Check sheet for the modelled part. Datum: model origin and axes. Units: mm. Coordinates: 2 decimals unless noted, no trailing zeros. Write each loop counter-clockwise with the first axis right and the second up, starting at its lowest first coordinate (ties: lowest second). Pieces come first, ordered by that corner, then holes. Notation, with made-up numbers: (-36, 71) - (20, 71) arc R20 cw to (20, 95) - close; hole circle Ø3 at (31.5, 89). An arc over 180 degrees is marked (long way). Use one line per item in the form item = value. Start each with the question number.
1. Cross-section at A-A on z = 15. Record the boundary of the cut face in (x, y) (3 decimals), then the cut area to 3 significant figures.
2. Cross-section at B-B on x = 12. Record the boundary of the cut face in (y, z).
3. Cross-section at D-D on y = 0.7. Give the number of separate pieces and of enclosed holes in the cut face, then the cut area to 3 significant figures.
4. Go/stop test with flat-tipped pins: pin 1 Ø4.5 at (x, z) = (-31, 0) entering from +Y; pin 2 Ø0.5 at (y, z) = (0.5, -0.5) entering from +X; pin 3 Ø0.5 at (y, z) = (0.5, -4) entering from -X; pin 4 Ø0.8 at (y, z) = (0.5, 3.5) entering from -X. Record where each tip stops, or that it passes through.
5. Scan lines: line 1 along X through (y, z) = (0.75, -15) (3 decimals); line 2 along X through (y, z) = (1.1, -7.5); line 3 along Z through (x, y) = (-4.5, 1.65). Record each from-to range of solid material in increasing order.
6. Cross-section at C-C on z = 0. Record the boundary of the cut face in (x, y) (3 decimals), then the cut area to 4 significant figures.
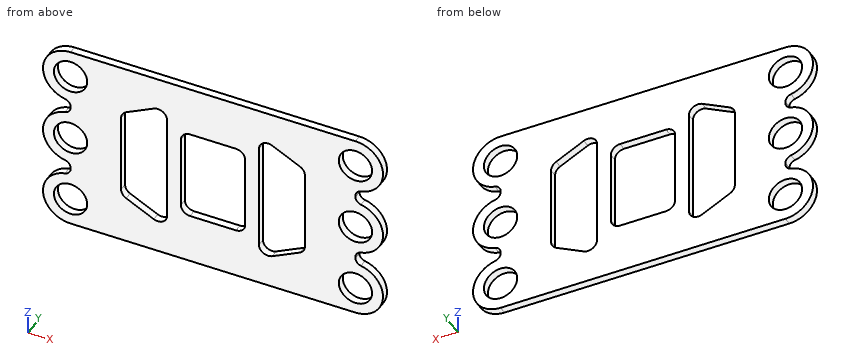
```python
from build123d import *

# Parameters (mm, degrees)
SKETCH1_R           = 6
SKETCH1_R_2         = 3.625
BOSS_EXTRUDE1_DEPTH = 1.7
CUT_EXTRUDE1_REACH  = 44.578
SKETCH2_W           = 10
SKETCH2_H           = 20
SKETCH2_W_2         = 14
FILLET1_R           = 1.5
FILLET2_R           = 2


with BuildPart() as part:
    # Sketch1 → Boss-Extrude1 (new body)
    # profile 1 of 7: a face of its own
    with BuildSketch(Plane(origin=(0, 0, 0), x_dir=(1, 0, 0), z_dir=(0, 1, 0))):
        with BuildLine():
            Line((31, 21), (-31, 21))
            ThreePointArc((-31, 21), (-26.757359313, 19.242640687), (-25, 15))
            ThreePointArc((-25, 15), (-26.757359313, 10.757359313), (-31, 9))
            Line((-31, 9), (-31, 6))
            ThreePointArc((-31, 6), (-26.757359313, 4.242640687), (-25, 0))
            ThreePointArc((-25, 0), (-26.757359313, -4.242640687), (-31, -6))
            Line((-31, -6), (-31, -9))
            ThreePointArc((-31, -9), (-26.757359313, -10.757359313), (-25, -15))
            ThreePointArc((-25, -15), (-26.757359313, -19.242640687), (-31, -21))
            Line((-31, -21), (31, -21))
            ThreePointArc((31, -21), (25, -15), (31, -9))
            Line((31, -9), (31, -6))
            ThreePointArc((31, -6), (25, 0), (31, 6))
            Line((31, 6), (31, 9))
            ThreePointArc((31, 9), (25, 15), (31, 21))
        make_face()
    # profile 2 of 7: a face of its own
    with BuildSketch(Plane(origin=(0, 0, 0), x_dir=(1, 0, 0), z_dir=(0, 1, 0))):
        with Locations((-31, 15)):
            Circle(SKETCH1_R)
        with Locations(Location((-31, 15, 0), (0, 0, 270))):
            Circle(SKETCH1_R_2, mode=Mode.SUBTRACT)
    # profile 3 of 7: a face of its own
    with BuildSketch(Plane(origin=(0, 0, 0), x_dir=(1, 0, 0), z_dir=(0, 1, 0))):
        with Locations((-31, 0)):
            Circle(SKETCH1_R)
        with Locations(Location((-31, 0, 0), (0, 0, 270))):
            Circle(SKETCH1_R_2, mode=Mode.SUBTRACT)
    # profile 4 of 7: a face of its own
    with BuildSketch(Plane(origin=(0, 0, 0), x_dir=(1, 0, 0), z_dir=(0, 1, 0))):
        with Locations((-31, -15)):
            Circle(SKETCH1_R)
        with Locations(Location((-31, -15, 0), (0, 0, 270))):
            Circle(SKETCH1_R_2, mode=Mode.SUBTRACT)
    # profile 5 of 7: a face of its own
    with BuildSketch(Plane(origin=(0, 0, 0), x_dir=(1, 0, 0), z_dir=(0, 1, 0))):
        with Locations((31, -15)):
            Circle(SKETCH1_R)
        with Locations(Location((31, -15, 0), (0, 0, 270))):
            Circle(SKETCH1_R_2, mode=Mode.SUBTRACT)
    # profile 6 of 7: a face of its own
    with BuildSketch(Plane(origin=(0, 0, 0), x_dir=(1, 0, 0), z_dir=(0, 1, 0))):
        with Locations((31, 0)):
            Circle(SKETCH1_R)
        with Locations(Location((31, 0, 0), (0, 0, 270))):
            Circle(SKETCH1_R_2, mode=Mode.SUBTRACT)
    # profile 7 of 7: a face of its own
    with BuildSketch(Plane(origin=(0, 0, 0), x_dir=(1, 0, 0), z_dir=(0, 1, 0))):
        with Locations((31, 15)):
            Circle(SKETCH1_R)
        with Locations(Location((31, 15, 0), (0, 0, 270))):
            Circle(SKETCH1_R_2, mode=Mode.SUBTRACT)
    extrude(amount=BOSS_EXTRUDE1_DEPTH)

    # Sketch2 → Cut-Extrude1 (cut, up to next)
    with BuildSketch(Plane(origin=(0, 1.7, 0), x_dir=(1, 0, 0), z_dir=(0, 1, 0)), mode=Mode.PRIVATE) as cut_extrude1_sk1:
        with Locations((-15, 0)):
            Rectangle(SKETCH2_W, SKETCH2_H)
    cut_extrude1_tool1 = extrude(cut_extrude1_sk1.sketch, amount=-CUT_EXTRUDE1_REACH, mode=Mode.PRIVATE) & part.part
    # Sketch2 → Cut-Extrude1 (cut, up to next)
    with BuildSketch(Plane(origin=(0, 1.7, 0), x_dir=(1, 0, 0), z_dir=(0, 1, 0)), mode=Mode.PRIVATE) as cut_extrude1_sk2:
        Polygon((-10, 10), (-10, 15), (-20, 10), align=None)
    cut_extrude1_tool2 = extrude(cut_extrude1_sk2.sketch, amount=-CUT_EXTRUDE1_REACH, mode=Mode.PRIVATE) & part.part
    # Sketch2 → Cut-Extrude1 (cut, up to next)
    with BuildSketch(Plane(origin=(0, 1.7, 0), x_dir=(1, 0, 0), z_dir=(0, 1, 0)), mode=Mode.PRIVATE) as cut_extrude1_sk3:
        Polygon((-10, -15), (-10, -10), (-20, -10), align=None)
    cut_extrude1_tool3 = extrude(cut_extrude1_sk3.sketch, amount=-CUT_EXTRUDE1_REACH, mode=Mode.PRIVATE) & part.part
    # Sketch2 → Cut-Extrude1 (cut, up to next)
    with BuildSketch(Plane(origin=(0, 1.7, 0), x_dir=(1, 0, 0), z_dir=(0, 1, 0)), mode=Mode.PRIVATE) as cut_extrude1_sk4:
        Polygon((10, -15), (20, -10), (10, -10), align=None)
    cut_extrude1_tool4 = extrude(cut_extrude1_sk4.sketch, amount=-CUT_EXTRUDE1_REACH, mode=Mode.PRIVATE) & part.part
    # Sketch2 → Cut-Extrude1 (cut, up to next)
    with BuildSketch(Plane(origin=(0, 1.7, 0), x_dir=(1, 0, 0), z_dir=(0, 1, 0)), mode=Mode.PRIVATE) as cut_extrude1_sk5:
        with Locations((15, 0)):
            Rectangle(SKETCH2_W, SKETCH2_H)
    cut_extrude1_tool5 = extrude(cut_extrude1_sk5.sketch, amount=-CUT_EXTRUDE1_REACH, mode=Mode.PRIVATE) & part.part
    # Sketch2 → Cut-Extrude1 (cut, up to next)
    with BuildSketch(Plane(origin=(0, 1.7, 0), x_dir=(1, 0, 0), z_dir=(0, 1, 0)), mode=Mode.PRIVATE) as cut_extrude1_sk6:
        Polygon((20, 10), (10, 15), (10, 10), align=None)
    cut_extrude1_tool6 = extrude(cut_extrude1_sk6.sketch, amount=-CUT_EXTRUDE1_REACH, mode=Mode.PRIVATE) & part.part
    # Sketch2 → Cut-Extrude1 (cut, up to next)
    with BuildSketch(Plane(origin=(0, 1.7, 0), x_dir=(1, 0, 0), z_dir=(0, 1, 0)), mode=Mode.PRIVATE) as cut_extrude1_sk7:
        Rectangle(SKETCH2_W_2, SKETCH2_H)
    cut_extrude1_tool7 = extrude(cut_extrude1_sk7.sketch, amount=-CUT_EXTRUDE1_REACH, mode=Mode.PRIVATE) & part.part
    add(cut_extrude1_tool1.solids().sort_by_distance((-15, 1.7, 0))[0], mode=Mode.SUBTRACT)
    add(cut_extrude1_tool2.solids().sort_by_distance((-13.333333, 1.7, -11.666667))[0], mode=Mode.SUBTRACT)
    add(cut_extrude1_tool3.solids().sort_by_distance((-13.333333, 1.7, 11.666667))[0], mode=Mode.SUBTRACT)
    add(cut_extrude1_tool4.solids().sort_by_distance((13.333333, 1.7, 11.666667))[0], mode=Mode.SUBTRACT)
    add(cut_extrude1_tool5.solids().sort_by_distance((15, 1.7, 0))[0], mode=Mode.SUBTRACT)
    add(cut_extrude1_tool6.solids().sort_by_distance((13.333333, 1.7, -11.666667))[0], mode=Mode.SUBTRACT)
    add(cut_extrude1_tool7.solids().sort_by_distance((0, 1.7, 0))[0], mode=Mode.SUBTRACT)

    # Fillet1
    fillet1_edges = [part.edges().sort_by_distance(p)[0] for p in [
        (31, 0.85, -9),
        (31, 0.85, -6),
        (31, 0.85, 6),
        (31, 0.85, 9),
        (-31, 0.85, 9),
        (-31, 0.85, 6),
        (-31, 0.85, -6),
        (-31, 0.85, -9),
    ]]
    fillet(fillet1_edges, radius=FILLET1_R)

    # Fillet2
    fillet2_edges = [part.edges().sort_by_distance(p)[0] for p in [
        (-20, 0.85, 10),
        (-20, 0.85, -10),
        (-10, 0.85, -15),
        (-10, 0.85, 15),
        (20, 0.85, 10),
        (10, 0.85, 15),
        (10, 0.85, -15),
        (20, 0.85, -10),
        (7, 0.85, -10),
        (7, 0.85, 10),
        (-7, 0.85, 10),
        (-7, 0.85, -10),
    ]]
    fillet(fillet2_edges, radius=FILLET2_R)


solid = part.part
```
Final values:
q1.outline = (-37, 0) - (-34.625, 0) - (-34.625, 1.7) - (-37, 1.7) - close; (-27.375, 0) - (27.375, 0) - (27.375, 1.7) - (-27.375, 1.7) - close; (34.625, 0) - (37, 0) - (37, 1.7) - (34.625, 1.7) - close
q1.area = 101 mm²
q2.outline = (0, -21) - (1.7, -21) - (1.7, -13.76) - (0, -13.76) - close; (0, 13.76) - (1.7, 13.76) - (1.7, 21) - (0, 21) - close
q3.separate_pieces = 1
q3.enclosed_holes = 9
q3.area = 1,930 mm²
q4.pin_1 = through
q4.pin_2 = 36.99
q4.pin_3 = -35.68
q4.pin_4 = -36.14
q5.line_1 = -37 to -34.625, -27.375 to 27.375, 34.625 to 37
q5.line_2 = -31 to -20, -10 to -7, 7 to 10, 20 to 31
q5.line_3 = -21 to -10, 10 to 21
q6.outline = (-37, 0) - (-34.625, 0) - (-34.625, 1.7) - (-37, 1.7) - close; (-27.375, 0) - (-20, 0) - (-20, 1.7) - (-27.375, 1.7) - close; (-10, 0) - (-7, 0) - (-7, 1.7) - (-10, 1.7) - close; (7, 0) - (10, 0) - (10, 1.7) - (7, 1.7) - close; (20, 0) - (27.375, 0) - (27.375, 1.7) - (20, 1.7) - close; (34.625, 0) - (37, 0) - (37, 1.7) - (34.625, 1.7) - close
q6.area = 43.35 mm²
